Work out the finished part from the listing and answer in its coordinate system (mm). A direction names the side the tool comes from. Round coordinates to 2 decimals unless told otherwise and drop trailing zeros. Loops run counter-clockwise (first coordinate to the right, second up) from the corner with the lowest first, then second, coordinate; pieces in that order, holes last.
from build123d import *

# Parameters (mm, degrees)
SKETCH1_W           = 35
SKETCH1_H           = 10
BOSS_EXTRUDE1_DEPTH = 10
SKETCH2_W           = 16
SKETCH2_H           = 10
BOSS_EXTRUDE2_DEPTH = 25
CUT_EXTRUDE3_START  = -7.959741
SKETCH3_R           = 4.1
CUT_EXTRUDE3_DEPTH  = 7.959741
SKETCH4_R           = 1.7
CUT_EXTRUDE4_DEPTH  = 13
SKETCH5_R           = 3
SKETCH5_R_2         = 1.7
CUT_EXTRUDE5_DEPTH  = 6
FILLET1_R           = 8


with BuildPart() as part:
    # Sketch1 → Boss-Extrude1 (new body)
    with BuildSketch(Plane.XY.offset(315.507646495)):
        with Locations((-0.05341426, 5.6352577)):
            Rectangle(SKETCH1_W, SKETCH1_H)
    extrude(amount=BOSS_EXTRUDE1_DEPTH)

    # Sketch2 → Boss-Extrude2 (add)
    with BuildSketch(Plane.XY.offset(325.507646495)):
        with Locations((-0.02670713, 5.6352577)):
            Rectangle(SKETCH2_W, SKETCH2_H)
    extrude(amount=BOSS_EXTRUDE2_DEPTH)

    # Sketch3 → Cut-Extrude3 (cut)
    with BuildSketch(Plane(origin=(0, 10.6352577, 0), x_dir=(1, 0, 0), z_dir=(0, 1, 0)).offset(CUT_EXTRUDE3_START)):
        with Locations(Location((-0.034055406, -340.877646495, 0), (0, 0, 270))):
            Circle(SKETCH3_R)
    extrude(amount=CUT_EXTRUDE3_DEPTH, mode=Mode.SUBTRACT)

    # Sketch4 → Cut-Extrude4 (cut)
    with BuildSketch(Plane.XY.offset(325.507646495)):
        with Locations((-12.790060695, 5.6352577)):
            Circle(SKETCH4_R)
        with Locations((12.709939305, 5.6352577)):
            Circle(SKETCH4_R)
    extrude(amount=-CUT_EXTRUDE4_DEPTH, mode=Mode.SUBTRACT)

    # Sketch5 → Cut-Extrude5 (cut)
    # profile 1 of 2: a face of its own
    with BuildSketch(Plane.XY.offset(325.507646495)):
        with Locations((-12.790060695, 5.6352577)):
            Circle(SKETCH5_R)
        with Locations((-12.790060695, 5.6352577)):
            Circle(SKETCH5_R_2, mode=Mode.SUBTRACT)
    # profile 2 of 2: a face of its own
    with BuildSketch(Plane.XY.offset(325.507646495)):
        with Locations((12.709939305, 5.6352577)):
            Circle(SKETCH5_R)
        with Locations((12.709939305, 5.6352577)):
            Circle(SKETCH5_R_2, mode=Mode.SUBTRACT)
    extrude(amount=-CUT_EXTRUDE5_DEPTH, mode=Mode.SUBTRACT)

    # Fillet1
    fillet1_edges = [part.edges().sort_by_distance(p)[0] for p in [
        (7.97329287, 5.6352577, 350.507646495),
        (-8.02670713, 5.6352577, 350.507646495),
    ]]
    fillet(fillet1_edges, radius=FILLET1_R - 0.0001)  # a hair under: the kernel refuses the full size


solid = part.part
Item 1: For faces 1 (the face through (0, 10.635, 329)), 2 (the face through (-8.027, 6, 334)), 3 (the face through (10.5, 7.9, 325.508)), 4 (the face through (0, 0.635, 329)), 5 (the face through (14, 4, 319.508)), determine the directions among +Z, -Z, +X, -X, +Y, -Y from which every point of the face is accessible in a straight line to the end or side of a thin tool.
Item 2: Section C-C, the plane z = 318 is taken. Give the vertices of the cut face in (x, y), plus the area to 3 significant figures.
Item 3: Section D-D, the plane z = 334.5 is taken. Give the vertices of the cut face in (x, y), plus the area to 3 significant figures.
Item 4: Section A-A, the plane x = -13.5 is taken. Give the vertices of the cut face in (y, z).
Item 5: Straight lines are drawn through the part: line 1 (X direction, y = 4.25, z = 341); line 2 (X direction, y = 2.5, z = 336.5); line 3 (Z direction, x = -12.5, y = 9.75). For each, find the intervals that lie inside material, in ascending order.
Item 6: Determine the mould class of faces 6 (the face through (-2.5, 6.6, 337.6)), 7 (the face through (0, 2.676, 341)), 8 (the face through (-15.17, 3.81, 322.55)), 9 (the face through (-15, 8, 325.508)) for opening direction Z: pulls with the +Z half, pulls with the -Z half, needs draft (parallel to the pull), parting line crosses it, or undercut.
Item 7: Each of these flat-tipped pins is pushed along its axis until it touches: P1, Ø2, axis at x = -12.79, y = 5.64, coming from the -Z side; P2, Ø3, axis at x = -12.5, y = 5, coming from the +Z side; P3, Ø2.5, axis at x = -1.5, z = 342, coming from the +Y side; P4, Ø5, axis at y = 8.5, z = 333.5, coming from the -X side. Where does it stop, or does it pass through?
Answer below:
1. face 1: +Z, -Z, +X, -X, +Y
1. face 2: +Z, -X, +Y, -Y
1. face 3: +Z, +X, +Y, -Y
1. face 4: +Z, -Z, +X, -X, -Y
1. face 5: +Z
2. outline: (-17.55, 0.64) - (17.45, 0.64) - (17.45, 10.64) - (-17.55, 10.64) - close; hole circle Ø3.4 at (-12.79, 5.64); hole circle Ø3.4 at (12.71, 5.64)
2. area: 332 mm2
3. outline: (-8.03, 0.64) - (7.97, 0.64) - (7.97, 10.64) - (-8.03, 10.64) - close
3. area: 160 mm2
4. outline: (0.64, 315.51) - (4.09, 315.51) - (4.09, 319.51) - (2.72, 319.51) - (2.72, 325.51) - (0.64, 325.51) - close; (7.18, 315.51) - (10.64, 315.51) - (10.64, 325.51) - (8.55, 325.51) - (8.55, 319.51) - (7.18, 319.51) - close
5. line 1: x = -8.03 to -4.13, 4.06 to 7.97
5. line 2: x = -8.03 to 7.97
5. line 3: z = 315.51 to 325.51
6. face 6: undercut
6. face 7: undercut
6. face 8: needs draft
6. face 9: pulls with the +Z half
7. P1: passes through
7. P2: stops at z = 319.51
7. P3: stops at y = 2.68
7. P4: stops at x = -8.03
